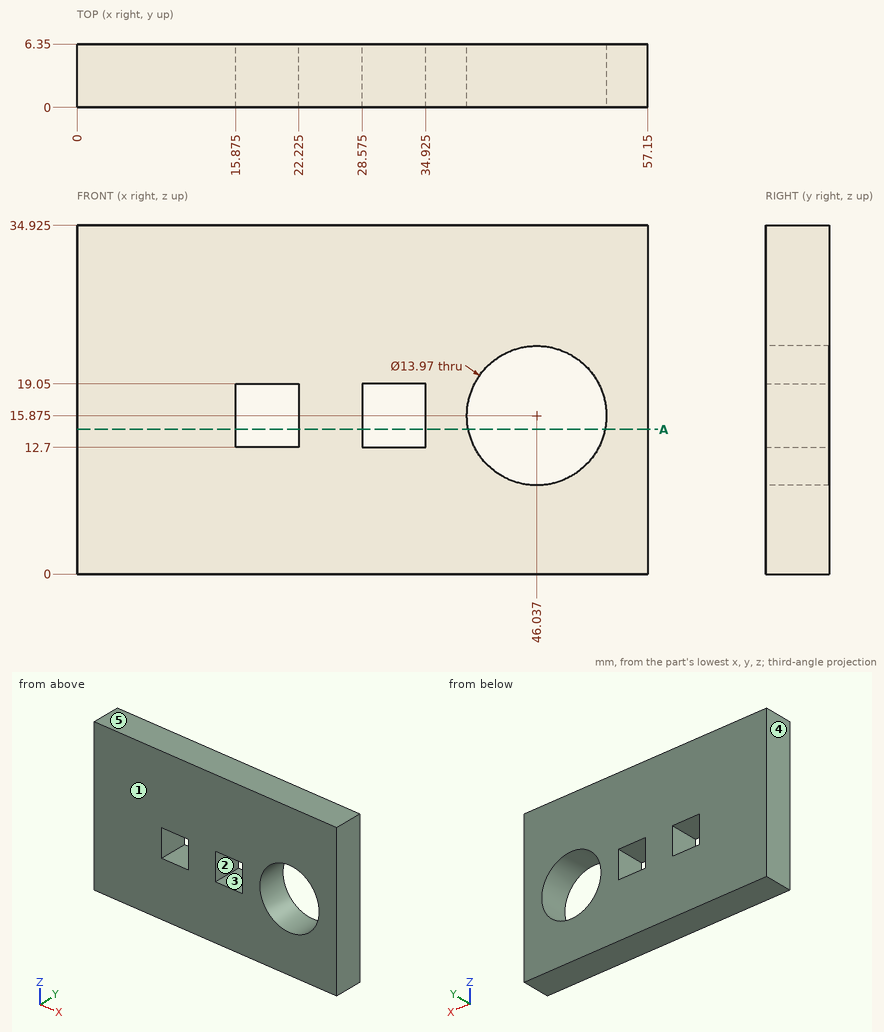
Answer from the drawing. Dimensions are ordinates in mm from the lowest x, y and z of the part. A direction names the side the tool comes from. Round coordinates to 2 decimals unless told otherwise and drop trailing zeros. Write each question's results on one line, items separated by ' | '. Start each with the question number.
Item 1: Find section A-A on z = 14.5. Give the number of separate pieces and of enclosed holes in the cut face, and give its area (3 significant figures).
Item 2: Which of the six approach directions +Z, -Z, +X, -X, +Y, -Y give full straight-line access (tool end or side, diameter ignored) to the marked faces 1 and 2?
Item 3: The mould has two halves that part along X. Classify the marked faces 3, 4 and 5: +X half, -X half, draft (parallel to the pull), parting line (faces both ways), or undercut.
Item 4: Given pin 1 Ø11 at (x, z) = (46.04, 15.88) entering from -Y, flat-ended and moving along its own axis, determine where the tip first touches the part or whether it passes through.
Item 5: A straight line is drawn through the part: probe 1 along Z at (x, y) = (51.5, 3.5) (1 decimal). Find the intervals that lie inside material, in ascending order.
Answer block:
1) separate pieces: 4 | enclosed holes: 0 | area: 195 mm²
2) face 1: +Z, -Z, +X, -X, -Y | face 2: +Y, -Y
3) face 3: undercut | face 4: -X half | face 5: draft
4) pin 1: passes through
5) probe 1: z = 0 to 11.5, 20.2 to 34.9
